Can you work these out from the model? Positions are in its coordinate system, mm. Face numbers are marked on the shaded views. Coordinates: 2 decimals unless noted, no trailing zeros. Order: outer loops, then holes, each group sorted by start corner. A loop starts at its lowest first (then second) coordinate and runs counter-clockwise, first axis right, second up. Notation, with made-up numbers: (76, -16) -> (130, -16) arc R29 ccw to (130, 21) -> close; hole circle Ø6 at (-38.5, -25.5). An arc over 180 degrees is marked (long way). Answer as CSV lines item,"result".
from build123d import *

# Parameters (mm, degrees)
F0_W     = 200
F0_H     = 200
F0_R     = 60
F1_DEPTH = 100
F2_SIZE  = 24
F4_DEPTH = 200


with BuildPart() as f1:
    # F0 (on Top) → F1 (new body, symmetric)
    with BuildSketch(Plane.XY):
        Rectangle(F0_W, F0_H)
        Circle(F0_R, mode=Mode.SUBTRACT)
    extrude(amount=F1_DEPTH, both=True)

    # F2
    f2_edges = [f1.edges().sort_by_distance(p)[0] for p in [
        (-100, -100, 0),
        (100, -100, 0),
        (100, 100, 0),
        (-100, 100, 0),
    ]]
    chamfer(f2_edges, length=F2_SIZE)

    # F3 (on face) → F4 (cut)
    with BuildSketch(Plane.XZ.offset(100)):
        Polygon((100, 45), (100, 100), (-76, 100), align=None)
    extrude(amount=-F4_DEPTH, mode=Mode.SUBTRACT)


solid = f1.part
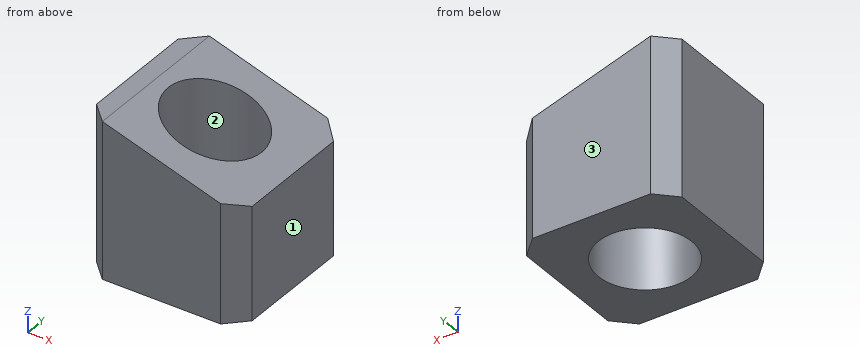
Q1. Imagine slicing it at B-B (x = 0). List the corners of the cut face in (y, z) for me.
Solution:
outline,"(-100, -100) -> (-60, -100) -> (-60, 76.25) -> (-100, 76.25) -> close; (60, -100) -> (100, -100) -> (100, 76.25) -> (60, 76.25) -> close"
Q2. Imagine slicing it at A-A (y = 0). List the corners of the cut face in (x, z) for me.
Solution:
outline,"(-100, -100) -> (-60, -100) -> (-60, 95) -> (-76, 100) -> (-100, 100) -> close; (60, -100) -> (100, -100) -> (100, 45) -> (60, 57.5) -> close"
Q3. We'd pull the mould along Y, two halves only. Please class the marked faces 1, 2 and 3: pulls with the +Y half, pulls with the -Y half, needs draft (parallel to the pull), parting line crosses it, or undercut.
Solution:
face 1,"needs draft"
face 2,"undercut"
face 3,"pulls with the +Y half"
Q4. Imagine slicing it at D-D (x = 33.5). List the corners of the cut face in (y, z) for me, and give its area (3 significant figures).
Solution:
outline,"(-100, -100) -> (-49.78, -100) -> (-49.78, 65.78) -> (-100, 65.78) -> close; (49.78, -100) -> (100, -100) -> (100, 65.78) -> (49.78, 65.78) -> close"
area,"16,700 mm2"
Q5. For P1, Ø8, axis at x = -38.5, y = -43, coming from the +Z side, with a flat end and sliding along its axis, tell me the tip position at first contact or that it passes through.
Solution:
P1,"z = 89.53"
Q6. If I drill on line 1 (Y direction, x = 0, z = -9); line 2 (Y direction, x = -55.5, z = -29), over which ranges is the centre line in solid material (lowest first)?
Solution:
line 1,"-100 to -60, 60 to 100"
line 2,"-100 to -22.8, 22.8 to 100"
Q7. Imagine slicing it at C-C (z = -58.5). List the corners of the cut face in (x, y) for me.
Solution:
outline,"(-100, -76) -> (-76, -100) -> (76, -100) -> (100, -76) -> (100, 76) -> (76, 100) -> (-76, 100) -> (-100, 76) -> close; hole circle Ø120 at (0, 0)"
